The listing builds one solid part. Answer for the finished solid, in the listing's coordinates (mm). Face numbers are marked on the shaded views. Give positions to 0.01 mm unless a question says otherwise; leave off trailing zeros. Write each loop counter-clockwise with the first axis right and the second up, starting at its lowest first coordinate (ties: lowest second). Pieces come first, ordered by that corner, then holes. Notation, with made-up numbers: (-8, 53) -> (-3, 53) arc R24 cw to (-3, 80) -> close; hole circle Ø1 at (68.25, 78.25). An arc over 180 degrees is marked (long way). Put each result on its own line as item: value. Start each with the question number.
1) A cutting plane is placed at D-D (y = 1.5). Write down the section's boundary in (x, z).
2) A cutting plane is placed at B-B (z = -2). Write down the section's boundary in (x, y).
3) Flat-ended cylindrical pins translate along their axes: pin 1 Ø1.5 at (x, z) = (5, -2.5) entering from +Y; pin 2 Ø1.3 at (x, z) = (0, 0) entering from +Y; pin 3 Ø2 at (x, z) = (15.5, 0.5) entering from -Y. Find the tip coordinate at first contact, or state that the pin passes through.
4) For a pull along Y with two mould halves and no side action, classify the marked faces 1, 2 and 3 as released by +Y, released by -Y, zero draft, split by the parting line, or undercut.
5) Find the intervals of material crossed by line 1 along Z through (x, y) = (0, -2.65) (3 decimals); line 2 along Z through (x, y) = (0, -0.6); line 3 along Y through (x, z) = (18, 1.5), in increasing order. Write a range as from..to.
6) A cutting plane is placed at A-A (z = 0). Write down the section's boundary in (x, y) (3 decimals).
7) A cutting plane is placed at C-C (x = 19.5). Write down the section's boundary in (y, z), then the cut area to 3 significant figures.
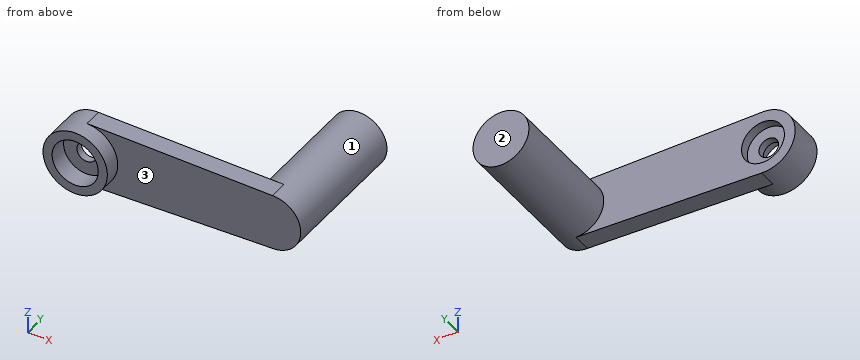
from build123d import *

# Parameters (mm, degrees)
ESBO_O1_R                = 3.45
RESSALTO_EXTRUS_O1_DEPTH = 1.4
ESBO_O2_R                = 3.45
RESSALTO_EXTRUS_O2_DEPTH = 2.4
FURO1_D                  = 4.95
FURO1_DEPTH              = 2
FURO2_D                  = 4.6
FURO2_DEPTH              = 1
FURO3_D                  = 2.1
BOSS_EXTRUDE1_DEPTH      = 2
SKETCH3_R                = 3
BOSS_EXTRUDE2_DEPTH      = 15


with BuildPart() as part:
    # Esboço1 → Ressalto-extrusão1 (new body)
    with BuildSketch(Plane(origin=(0, 0, 0), x_dir=(1, 0, 0), z_dir=(0, 1, 0))):
        with Locations(Location((0, 0, 0), (0, 0, 270))):
            Circle(ESBO_O1_R)
    extrude(amount=-RESSALTO_EXTRUS_O1_DEPTH)

    # Esboço2 → Ressalto-extrusão2 (add)
    with BuildSketch(Plane.XZ.offset(1.4)):
        with Locations(Location((0, 0, 0), (0, 0, 90))):
            Circle(ESBO_O2_R)
    extrude(amount=RESSALTO_EXTRUS_O2_DEPTH)

    # Furo1
    with Locations(Plane(origin=(0, -3.8, 0), x_dir=(-1, 0, 0), z_dir=(0, -1, 0))):
        with Locations((0, 0)):
            Hole(FURO1_D / 2, depth=FURO1_DEPTH)

    # Furo2
    with Locations(Plane(origin=(0, 0, 0), x_dir=(1, 0, 0), z_dir=(0, 1, 0))):
        with Locations((0, 0)):
            Hole(FURO2_D / 2, depth=FURO2_DEPTH)

    # Furo3 (through all)
    with Locations(Plane(origin=(0, 0, 0), x_dir=(1, 0, 0), z_dir=(0, 1, 0))):
        with Locations((0, 0)):
            Hole(FURO3_D / 2)

    # Sketch2 → Boss-Extrude1 (add)
    with BuildSketch(Plane(origin=(0, 0, 0), x_dir=(1, 0, 0), z_dir=(0, 1, 0))):
        with BuildLine():
            Line((20.067369497, 2.999243463), (0.154910769, 3.446520369))
            ThreePointArc((0.154910769, 3.446520369), (2.493686243, 2.384120157), (3.45, 0))
            ThreePointArc((3.45, 0), (2.493686243, -2.384120157), (0.154910769, -3.446520369))
            Line((0.154910769, -3.446520369), (20.067369497, -2.999243463))
            ThreePointArc((20.067369497, -2.999243463), (23, 0), (20.067369497, 2.999243463))
        make_face()
    extrude(amount=-BOSS_EXTRUDE1_DEPTH)

    # Sketch3 → Boss-Extrude2 (add)
    with BuildSketch(Plane.XZ.offset(2)):
        with Locations(Location((20.067369497, 0, 0), (0, 0, 270))):
            Circle(SKETCH3_R)
    extrude(amount=-BOSS_EXTRUDE2_DEPTH)


solid = part.part
Reply:
1. outline: circle Ø6 at (20.07, 0)
2. outline: (-2.81, -3.8) -> (-1.46, -3.8) -> (-1.46, -1.8) -> (1.46, -1.8) -> (1.46, -3.8) -> (2.81, -3.8) -> (2.81, -2) -> (22.3, -2) -> (22.3, 13) -> (17.83, 13) -> (17.83, 0) -> (1.14, 0) -> (1.14, -1) -> (-1.14, -1) -> (-1.14, 0) -> (-2.81, 0) -> close
3. pin 1: stops at y = 0
3. pin 2: passes through
3. pin 3: stops at y = -2
4. face 1: zero draft
4. face 2: released by +Y
4. face 3: released by -Y
5. line 1: z = -3.45..-2.475, 2.475..3.45
5. line 2: z = -3.45..-2.3, 2.3..3.45
5. line 3: y = -2..13
6. outline: (-3.45, -3.8) -> (-2.475, -3.8) -> (-2.475, -1.8) -> (-1.05, -1.8) -> (-1.05, -1) -> (-2.3, -1) -> (-2.3, 0) -> (-3.45, 0) -> close; (1.05, -1.8) -> (2.475, -1.8) -> (2.475, -3.8) -> (3.45, -3.8) -> (3.45, -2) -> (23.067, -2) -> (23.067, 13) -> (17.067, 13) -> (17.067, 0) -> (2.3, 0) -> (2.3, -1) -> (1.05, -1) -> close
7. outline: (-2, -3.01) -> (0, -3.01) -> (0, -2.95) -> (13, -2.95) -> (13, 2.95) -> (0, 2.95) -> (0, 3.01) -> (-2, 3.01) -> close
7. area: 88.6 mm2
